Geometry check sheet. Reference: the model listing, model coordinates, mm. Coordinates: 2 decimals unless noted, no trailing zeros. Write each loop counter-clockwise with the first axis right and the second up, starting at its lowest first coordinate (ties: lowest second). Pieces come first, ordered by that corner, then holes. Notation, with made-up numbers: (87.25, -24.5) -> (146.25, -24.5) arc R31 ccw to (146.25, 11.5) -> close; hole circle Ø8 at (39.5, -40). An arc over 180 degrees is marked (long way). One line per question, with ' | ' between items.
from build123d import *

# Parameters (mm, degrees)
F0_R     = 12.5
F1_DEPTH = 25
F2_DEPTH = 12.5
F4_R     = 7.5
F6_R     = 6
F7_DEPTH = 37.5010001


with BuildPart() as f1:
    # F0 (on Top) → F1 (new body)
    with BuildSketch(Plane.XY):
        Circle(F0_R)
    extrude(amount=F1_DEPTH)



with BuildPart() as f2:
    # F0 (on Top) → F2 (new body, symmetric)
    with BuildSketch(Plane.XY):
        with Locations((150, 0)):
            Circle(F0_R)
    extrude(amount=F2_DEPTH, both=True)


with BuildPart() as f1_1:
    add(f1.part)

    add(f2.part)  # F5 merges F2
    # F5: sweep along a path in F3
    with BuildLine(Plane.XZ) as f5_path:
        Line((0, 12.5), (25, 12.5))
        ThreePointArc((25, 12.5), (32.4420840754, 12.0366726028), (39.7692307692, 10.6538461538))
        ThreePointArc((39.7692307692, 10.6538461538), (82.0529731485, 2.6737851879), (125, 0))
        Line((125, 0), (150, 0))
    # F4 (on Right) → F5 (sweep)
    with BuildSketch(Plane.YZ):
        with Locations((0, 12.5)):
            Circle(F4_R)
    sweep(path=f5_path.line)

    # F6 (on face) → F7 (cut, through all)
    with BuildSketch(Plane.XY.offset(25)):
        Circle(F6_R)
        with Locations((150, 0)):
            Circle(F6_R)
    extrude(amount=-F7_DEPTH, mode=Mode.SUBTRACT)


solid = f1_1.part
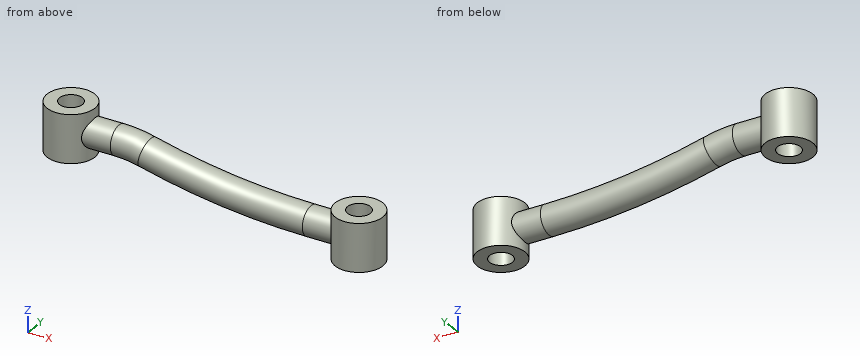
1. Material ranges on line 1 (Y direction, x = 0, z = 7); line 2 (Y direction, x = 42.5, z = 10.5); line 3 (X direction, y = -2.5, z = -11), recorded low to high. Write a range as from..to.
Worked answers:
line 1: -12.5..-6, 6..12.5 | line 2: -7.48..7.48 | line 3: 137.75..144.55, 155.45..162.25
2. Cross-section at B-B on x = 150. Record the boundary of the cut face in (y, z).
Worked answers:
outline: (-12.5, -12.5) -> (-6, -12.5) -> (-6, 12.5) -> (-12.5, 12.5) -> close; (6, -12.5) -> (12.5, -12.5) -> (12.5, 12.5) -> (6, 12.5) -> close
3. Cross-section at C-C on x = 128.5. Record the boundary of the cut face in (y, z).
Worked answers:
outline: circle Ø15 at (0, 0)
4. Cross-section at A-A on y = 0. Record the boundary of the cut face in (x, z), and give its area (3 significant figures).
Worked answers:
outline: (-12.5, 0) -> (-6, 0) -> (-6, 25) -> (-12.5, 25) -> close; (6, 0) -> (12.5, 0) -> (12.5, 5) -> (25, 5) arc R52.5 cw to (37.92, 3.38) arc R353.75 ccw to (125, -7.5) -> (137.5, -7.5) -> (137.5, -12.5) -> (144, -12.5) -> (144, 12.5) -> (137.5, 12.5) -> (137.5, 7.5) -> (125, 7.5) arc R338.75 cw to (41.62, 17.92) arc R67.5 ccw to (25, 20) -> (12.5, 20) -> (12.5, 25) -> (6, 25) -> close; (156, -12.5) -> (162.5, -12.5) -> (162.5, 12.5) -> (156, 12.5) -> close | area: 2,540 mm²
5. Go/stop test with flat-tipped pins: P1, Ø2, axis at x = 50, z = 8.5, coming from the +Y side; P2, Ø4, axis at y = -9.5, z = -7, coming from the -X side; P3, Ø6, axis at x = 65, y = 8.5, coming from the +Z side. Record where each tip stops, or that it passes through.
Worked answers:
P1: y = 7.5 | P2: x = 140 | P3: z = 10.46
